Read the model definition and answer for the solid it produces. Units are mm, in the model's axes. A direction names the side the tool comes from. Round coordinates to 2 decimals unless told otherwise and drop trailing zeros. Loops run counter-clockwise (first coordinate to the right, second up) from the corner with the lowest first, then second, coordinate; pieces in that order, holes last. Notation, with made-up numbers: (49.25, -26) -> (106.25, -26) arc R30 cw to (106.25, 0) -> close; hole circle Ø6 at (1.5, 7.5). An arc over 180 degrees is marked (long way). Put each result on its own line as item: value.
from build123d import *

# Parameters (mm, degrees)
SKETCH_222_W              = 2.54
SKETCH_222_H              = 2.4
EXTRUDE_699_DEPTH         = 6.7
EXTRUDE_699_DEPTH_BACK    = 0.4
SKETCH_753_W              = 2.54
SKETCH_753_H              = 0.75
EXTRUDE_1132_DEPTH        = 0.4
SKETCH_1186_W             = 2.54
SKETCH_1186_H             = 2.4
SKETCH_1186_W_2           = 0.9
SKETCH_1186_H_2           = 0.9
EXTRUDE_1471_DEPTH        = 0.8
CHAMFER_1532_SIZE         = 0.6
PATTERN_LINEAR_1658_COUNT = 8
PATTERN_LINEAR_1658_PITCH = 2.54
EXTRUDE_1_DEPTH           = 0.64
EXTRUDE_START             = -20.96
EXTRUDE_2_DEPTH           = 0.64


with BuildPart() as part:
    # Sketch 222 → Extrude 699 (new body, two sides)
    with BuildSketch(Plane.XY) as extrude_699_sk:
        Rectangle(SKETCH_222_W, SKETCH_222_H)
        Polygon((-1, 0.35), (-0.45, 0.35), (-0.45, 0.45), (0.45, 0.45), (0.45, 0.35), (1, 0.35), (1, -0.35), (0.45, -0.35), (0.45, -0.45), (-0.45, -0.45), (-0.45, -0.35), (-1, -0.35), align=None, mode=Mode.SUBTRACT)
    extrude(amount=EXTRUDE_699_DEPTH)
    extrude(extrude_699_sk.sketch, amount=-EXTRUDE_699_DEPTH_BACK)

    # Sketch 753 → Extrude 1132 (add)
    with BuildSketch(Plane(origin=(0, 0, -0.4), x_dir=(-1, 0, 0), z_dir=(0, 0, -1))):
        with Locations((0, -0.825)):
            Rectangle(SKETCH_753_W, SKETCH_753_H)
        with Locations((0, 0.825)):
            Rectangle(SKETCH_753_W, SKETCH_753_H)
    extrude(amount=EXTRUDE_1132_DEPTH)

    # Sketch 1186 → Extrude 1471 (add)
    with BuildSketch(Plane.XY.offset(6.7)):
        Rectangle(SKETCH_1186_W, SKETCH_1186_H)
        Rectangle(SKETCH_1186_W_2, SKETCH_1186_H_2, mode=Mode.SUBTRACT)
    extrude(amount=EXTRUDE_1471_DEPTH)

    # Chamfer 1532
    chamfer_1532_edges = [part.edges().sort_by_distance(p)[0] for p in [
        (0.45, 0, 7.5),
        (0, 0.45, 7.5),
        (-0.45, 0, 7.5),
        (0, -0.45, 7.5),
    ]]
    chamfer(chamfer_1532_edges, length=CHAMFER_1532_SIZE)


with BuildPart() as pattern_linear_1658_1:
    # Pattern Linear 1658: pattern copy
    add(part.part.moved(Location(Vector(-1, 0, 0) * (1 * PATTERN_LINEAR_1658_PITCH))))


with BuildPart() as pattern_linear_1658_2:
    # Pattern Linear 1658: pattern copy
    add(part.part.moved(Location(Vector(-1, 0, 0) * (2 * PATTERN_LINEAR_1658_PITCH))))


with BuildPart() as pattern_linear_1658_3:
    # Pattern Linear 1658: pattern copy
    add(part.part.moved(Location(Vector(-1, 0, 0) * (3 * PATTERN_LINEAR_1658_PITCH))))


with BuildPart() as pattern_linear_1658_4:
    # Pattern Linear 1658: pattern copy
    add(part.part.moved(Location(Vector(-1, 0, 0) * (4 * PATTERN_LINEAR_1658_PITCH))))


with BuildPart() as pattern_linear_1658_5:
    # Pattern Linear 1658: pattern copy
    add(part.part.moved(Location(Vector(-1, 0, 0) * (5 * PATTERN_LINEAR_1658_PITCH))))


with BuildPart() as pattern_linear_1658_6:
    # Pattern Linear 1658: pattern copy
    add(part.part.moved(Location(Vector(-1, 0, 0) * (6 * PATTERN_LINEAR_1658_PITCH))))


with BuildPart() as pattern_linear_1658_7:
    # Pattern Linear 1658: pattern copy
    add(part.part.moved(Location(Vector(-1, 0, 0) * (7 * PATTERN_LINEAR_1658_PITCH))))


with BuildPart() as part_1:
    add(part.part)

    # Combine 1774: union Pattern Linear 1658_7, Pattern Linear 1658_6, Pattern Linear 1658_5, Pattern Linear 1658_4, Pattern Linear 1658_3, Pattern Linear 1658_2, Pattern Linear 1658_1
    add(pattern_linear_1658_7.part)
    add(pattern_linear_1658_6.part)
    add(pattern_linear_1658_5.part)
    add(pattern_linear_1658_4.part)
    add(pattern_linear_1658_3.part)
    add(pattern_linear_1658_2.part)
    add(pattern_linear_1658_1.part)

    # Sketch 2582 → Бобышка-БоковаяНакладка1 (add)
    with BuildSketch(Plane(origin=(1.27, 0, 0), x_dir=(0, 0, -1), z_dir=(1, 0, 0))):
        Polygon((0.8, 1.2), (0.8, 0.45), (0.4, 0.45), (0.4, -0.45), (0.8, -0.45), (0.8, -1.2), (-7.5, -1.2), (-7.5, 1.2), align=None)
    extrude(amount=EXTRUDE_1_DEPTH)

    # Эскиз-БоковаяНакладка<2> → Бобышка-БоковаяНакладка2 (add)
    with BuildSketch(Plane(origin=(1.27, 0, 0), x_dir=(0, 0, -1), z_dir=(1, 0, 0)).offset(EXTRUDE_START)):
        Polygon((0.8, 1.2), (0.8, 0.45), (0.4, 0.45), (0.4, -0.45), (0.8, -0.45), (0.8, -1.2), (-7.5, -1.2), (-7.5, 1.2), align=None)
    extrude(amount=EXTRUDE_2_DEPTH)


solid = part_1.part
Item 1: The part is cut by section B-B (z = 4.25). State how many separate pieces and enclosed holes the cut face has, then the cut area to 3 significant figures.
Derived:
separate pieces: 1
enclosed holes: 8
area: 39.2 mm^2
Item 2: The part is cut by section A-A (x = 0). Determine the outline of the cut face in (y, z).
Derived:
outline: (-1.2, -0.8) -> (-0.45, -0.8) -> (-0.45, 6.9) -> (-1.05, 7.5) -> (-1.2, 7.5) -> close; (0.45, -0.8) -> (1.2, -0.8) -> (1.2, 7.5) -> (1.05, 7.5) -> (0.45, 6.9) -> close
Item 3: A flat-ended cylindrical pin translates along its axis: pin 1 Ø0.7 at (x, y) = (1, 0) entering from -Z. Find the tip coordinate at first contact, or state that the pin passes through.
Derived:
pin 1: stops at z = -0.4
Item 4: Which of the six approach directions +Z, -Z, +X, -X, +Y, -Y give full straight-line access (tool end or side, diameter ignored) to faces 4 (the flat face through (-16.5, 0, -0.4)), 5 (the flat face through (1.91, 0, 3))?
Derived:
face 4: -Z, +X, -X
face 5: +Z, -Z, +X, +Y, -Y
Item 5: Find the intervals of material crossed by line 1 along Y through (x, z) = (-10.5, -0.5); line 2 along Z through (x, y) = (-1.5, -0.35), in increasing order.
Derived:
line 1: y = -1.2 to -0.45, 0.45 to 1.2
line 2: z = -0.4 to 7.49
Item 6: For a pull along Y with two mould halves and no side action, classify faces 1 (the flat face through (-19.69, 0, 3)), 2 (the flat face through (-19, 0, -0.4)), 3 (the flat face through (-9, 1.2, 3)) as pulls with the +Y half, pulls with the -Y half, needs draft (parallel to the pull), parting line crosses it, or undercut.
Derived:
face 1: needs draft
face 2: undercut
face 3: pulls with the +Y half
